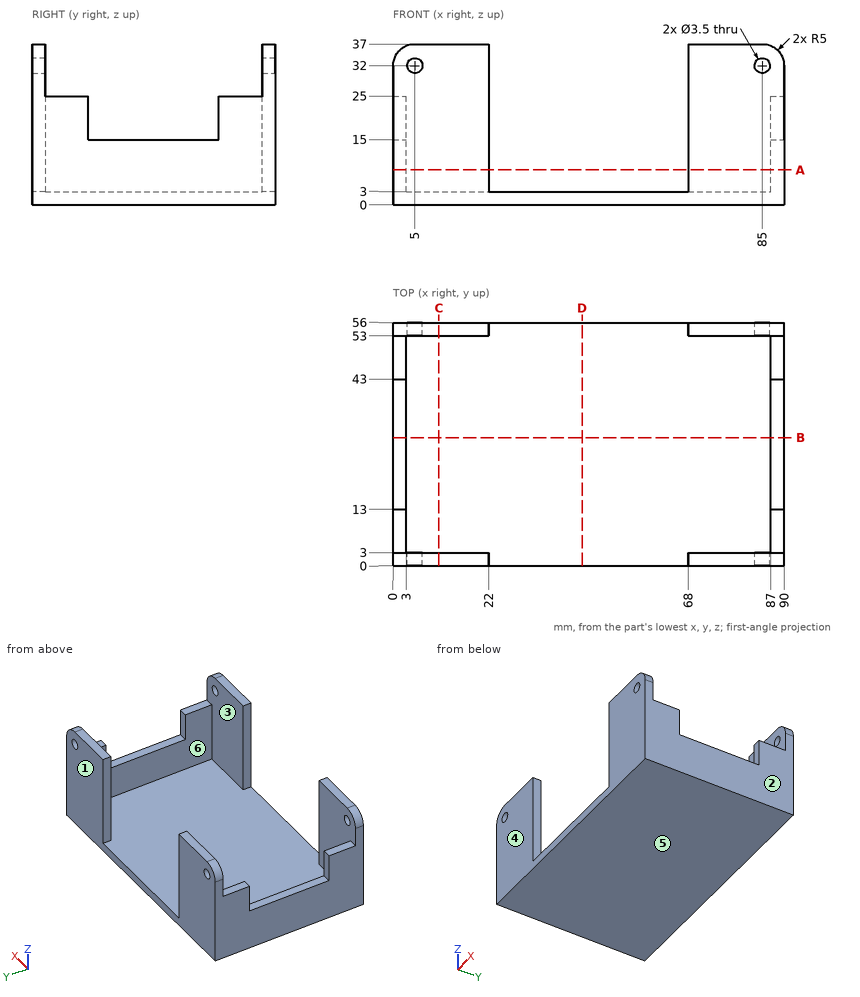
Study the drawing (mm; zero at the part's minimum x, y, z) and answer. A direction names the side the tool comes from. Coordinates: 2 decimals unless noted, no trailing zeros. Write each loop counter-clockwise with the first axis right and the second up, starting at its lowest first coordinate (ties: lowest second). Pieces come first, ordered by that corner, then holes.
Q1. Find the intervals of material crossed by line 1 along X through (y, z) = (53.95, 32); line 2 along Y through (x, z) = (10.5, 21); line 3 along X through (y, z) = (14.5, 8), in increasing order.
Returned:
line 1: x = 0 to 3.25, 6.75 to 22, 68 to 83.25, 86.75 to 90
line 2: y = 0 to 3, 53 to 56
line 3: x = 0 to 3, 87 to 90
Q2. Given P1, Ø3.5, axis at x = 89, y = 10, coming from the +Z side; P2, Ø3.5, axis at x = 88, y = 29.5, coming from the +Z side; P3, Ø12, axis at x = 24.5, y = 42.5, coming from the +Z side, each flat-ended and moving along its own axis, determine where each tip first touches the part or whether it passes through.
Returned:
P1: stops at z = 25
P2: stops at z = 15
P3: stops at z = 3
Q3. Section D-D, the plane x = 43.5 is taken. Write down the section's boundary in (y, z).
Returned:
outline: (0, 0) - (56, 0) - (56, 3) - (0, 3) - close
Q4. Section A-A, the plane z = 8 is taken. Write down the section's boundary in (x, y), then the cut area to 3 significant figures.
Returned:
outline: (0, 0) - (22, 0) - (22, 3) - (3, 3) - (3, 53) - (22, 53) - (22, 56) - (0, 56) - close; (68, 0) - (90, 0) - (90, 56) - (68, 56) - (68, 53) - (87, 53) - (87, 3) - (68, 3) - close
area: 564 mm2
Q5. Which of the six approach directions +Z, -Z, +X, -X, +Y, -Y give full straight-line access (tool end or side, diameter ignored) to the marked faces 5 and 6?
Returned:
face 5: -Z, +X, -X, +Y, -Y
face 6: +Z
Q6. The mould has two halves that part along Y. Classify the marked faces 1, 2, 3 and 4: released by +Y, released by -Y, zero draft, split by the parting line, or undercut.
Returned:
face 1: released by +Y
face 2: zero draft
face 3: undercut
face 4: released by -Y
Q7. Section B-B, the plane y = 29.5 is taken. Write down the section's boundary in (x, z).
Returned:
outline: (0, 0) - (90, 0) - (90, 15) - (87, 15) - (87, 3) - (3, 3) - (3, 15) - (0, 15) - close
Q8. Section C-C, the plane x = 10.5 is taken. Write down the section's boundary in (y, z).
Returned:
outline: (0, 0) - (56, 0) - (56, 37) - (53, 37) - (53, 3) - (3, 3) - (3, 37) - (0, 37) - close
